Solid Edge part; units mm, degrees
sketch "Sketch1" plane through (0, 0, 0) normal (0, 0, 1) x (1, 0, 0)
  line L0 (7.9, 5.2) -> (7.9, 12.5)
  line L1 (0, 12.5) -> (7.9, 12.5)
  line L2 (0, 0) -> (0, 12.5)
  line L3 (0, 0) -> (11.3, 0)
  line L4 (11.3, 0) -> (11.3, 5.2)
  line L5 (11.3, 5.2) -> (7.9, 5.2)
extrude "Protrusion1" add sketch "Sketch1" against normal blind 31.5
hole "Hole_1" at (4, 12.5, -25.5) direction (0, -1, 0) diameter 4 depth 6
hole "Hole1" at (4, 12.5, -6) direction (0, -1, 0) diameter 4 depth 6
Source: CAD feature listing. Evaluate the final solid. Frame: model axes, mm. A direction names the side the tool comes from. Coordinates: 2 decimals unless noted, no trailing zeros. Write each loop counter-clockwise with the first axis right and the second up, starting at its lowest first coordinate (ties: lowest second). Pieces come first, ordered by that corner, then holes. Notation, with made-up numbers: (59.5, 11.5) -> (95.5, 11.5) arc R19 cw to (95.5, 36.5) -> close; hole circle Ø4 at (77, 1.5). An arc over 180 degrees is marked (long way). Return JSON: item names as keys, results as strings. Group by question number.
1) Section query B-B, the plane y = 9. Return loops of the section in (x, z), plus the area to 3 significant figures.
2) Section query D-D, the plane z = -3. Return loops of the section in (x, y).
3) Section query A-A, the plane z = -25.5. Return loops of the section in (x, y).
4) Set-up query: faces 4 (the face through (4, 6, -31.5)), 5 (the face through (10, 5.2, -16)), 6 (the face through (4, 6.5, -26)). Return all of +Z, -Z, +X, -X, +Y, -Y with unobstructed straight access to the full face (end or side cutting, diameter ignored); none if empty.
5) Contact query for flat-ended pins moving along their axis: P1, Ø3, axis at y = 10, z = -24, coming from the +X side; P2, Ø4.5, axis at x = 4.5, z = -6.5, coming from the +Y side; P3, Ø1, axis at x = 9, z = -18, coming from the +Y side; P4, Ø3.5, axis at x = 4, z = -6, coming from the +Y side. Output: stop coordinate, or through.
6) Section query C-C, the plane x = 2.5. Return loops of the section in (y, z).
7) Ray query, line 1 along Z through (x, y) = (4, 7.95); line 2 along X through (y, z) = (8.65, -6); line 3 along X through (y, z) = (9.75, -23). Return the intervals inside material, ascending.
8) Mould query, pull axis Z, two halves, no side actions, for faces 1 (the face through (4, 6, 0)), 2 (the face through (3.912, 9.458, -27.498)), 3 (the face through (0, 6, -16)). Classes: +Z half, -Z half, draft (parallel to the pull), parting line (faces both ways), or undercut.
From the geometry:
{
 "1": {"outline": "(0, -31.5) -> (7.9, -31.5) -> (7.9, 0) -> (0, 0) -> close; hole circle Ø4 at (4, -25.5); hole circle Ø4 at (4, -6)", "area": "224 mm²"},
 "2": {"outline": "(0, 0) -> (11.3, 0) -> (11.3, 5.2) -> (7.9, 5.2) -> (7.9, 12.5) -> (0, 12.5) -> close"},
 "3": {"outline": "(0, 0) -> (11.3, 0) -> (11.3, 5.2) -> (7.9, 5.2) -> (7.9, 12.5) -> (6, 12.5) -> (6, 6.5) -> (2, 6.5) -> (2, 12.5) -> (0, 12.5) -> close"},
 "4": {"face 4": "-Z, +X, -X, +Y, -Y", "face 5": "+Z, -Z, +X, +Y", "face 6": "+Y"},
 "5": {"P1": "x = 7.9", "P2": "y = 12.5", "P3": "y = 5.2", "P4": "y = 6.5"},
 "6": {"outline": "(0, -31.5) -> (12.5, -31.5) -> (12.5, -26.82) -> (6.5, -26.82) -> (6.5, -24.18) -> (12.5, -24.18) -> (12.5, -7.32) -> (6.5, -7.32) -> (6.5, -4.68) -> (12.5, -4.68) -> (12.5, 0) -> (0, 0) -> close"},
 "7": {"line 1": "-31.5 to -27.5, -23.5 to -8, -4 to 0", "line 2": "0 to 2, 6 to 7.9", "line 3": "0 to 7.9"},
 "8": {"face 1": "+Z half", "face 2": "undercut", "face 3": "draft"}
}
